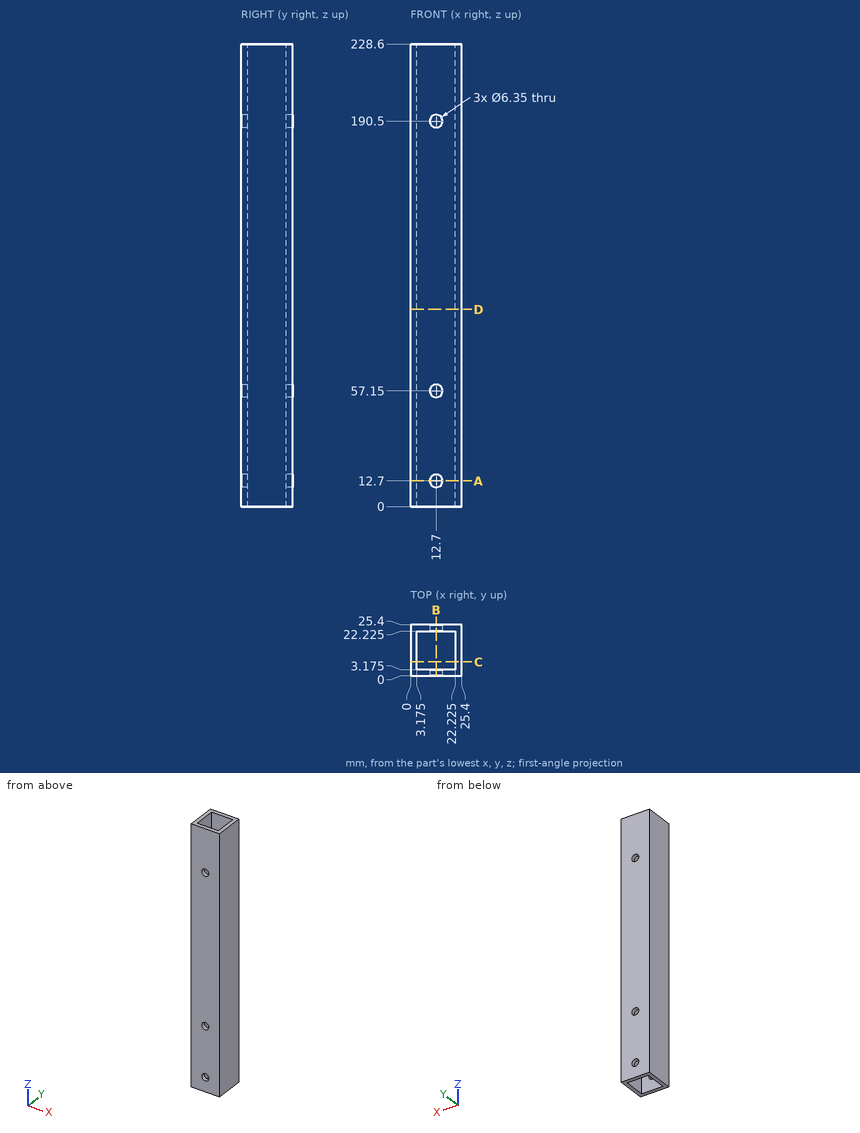
Geometry check sheet. Reference: drawing and pictorial views, mm from the part's lowest x, y, z. Coordinates: 2 decimals unless noted, no trailing zeros. Order: outer loops, then holes, each group sorted by start corner. A loop starts at its lowest first (then second) coordinate and runs counter-clockwise, first axis right, second up. Notation, with made-up numbers: (33, 55.25) - (79, 55.25) arc R13 cw to (79, 73.25) - close; hole circle Ø10 at (20.25, 26). An arc over 180 degrees is marked (long way). Answer in a Markdown table with one row per item. Add a question column.
1) Material ranges on line 1 along Z through (x, y) = (12.7, 2.4) (3 decimals); line 2 along X through (y, z) = (3.75, 152.5) (3 decimals), recorded low to high. Write a range as [from, to].
2) Cross-section at D-D, the plane z = 97.5. Record the cut outline in (x, y) (3 decimals).
3) Gauge pin test, flat end, axial feed: P1, Ø9.5, axis at x = 12.5, z = 80.5, coming from the -Y side. Record the tip position at first contact, or that the pin passes through.
4) Cross-section at A-A, the plane z = 12.7. Record the cut outline in (x, y) (3 decimals), then the cut area to 3 significant figures.
5) Cross-section at B-B, the plane x = 12.7. State how many separate pieces and enclosed holes the cut face has, then the cut area to 3 significant figures.
6) Cross-section at C-C, the plane y = 7. Record the cut outline in (x, z) (3 decimals).
Check result:
| question | item | result |
|---|---|---|
| 1 | line 1 | z = [0, 9.525], [15.875, 53.975], [60.325, 187.325], [193.675, 228.6] |
| 1 | line 2 | x = [0, 3.175], [22.225, 25.4] |
| 2 | outline | (0, 0) - (25.4, 0) - (25.4, 25.4) - (0, 25.4) - close; hole (3.175, 3.175) - (22.225, 3.175) - (22.225, 22.225) - (3.175, 22.225) - close |
| 3 | P1 | stops at y = 0 |
| 4 | outline | (0, 0) - (9.525, 0) - (9.525, 3.175) - (3.175, 3.175) - (3.175, 22.225) - (9.525, 22.225) - (9.525, 25.4) - (0, 25.4) - close; (15.875, 0) - (25.4, 0) - (25.4, 25.4) - (15.875, 25.4) - (15.875, 22.225) - (22.225, 22.225) - (22.225, 3.175) - (15.875, 3.175) - close |
| 4 | area | 242 mm² |
| 5 | separate pieces | 8 |
| 5 | enclosed holes | 0 |
| 5 | area | 1,330 mm² |
| 6 | outline | (0, 0) - (3.175, 0) - (3.175, 228.6) - (0, 228.6) - close; (22.225, 0) - (25.4, 0) - (25.4, 228.6) - (22.225, 228.6) - close |
